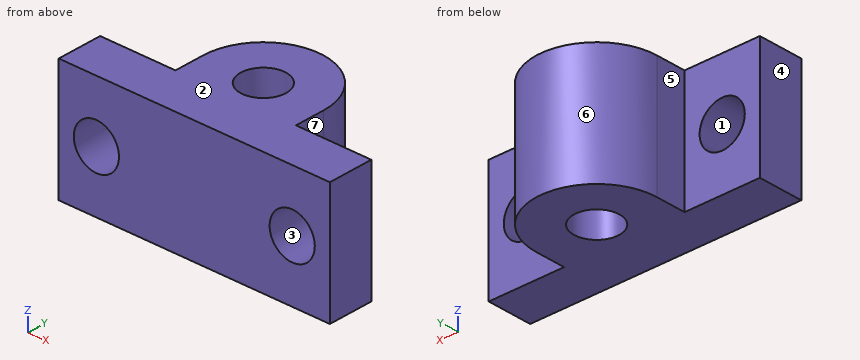
```python
from build123d import *

# Parameters (mm, degrees)
BOSS_EXTRUDE1_DEPTH = 8
SKETCH2_W           = 8
SKETCH2_H           = 3
BOSS_EXTRUDE2_DEPTH = 5
CUT_EXTRUDE1_REACH  = 18.401
SKETCH3_R           = 1.5
SKETCH4_W           = 8
SKETCH4_H           = 3
BOSS_EXTRUDE3_DEPTH = 5
CUT_EXTRUDE2_REACH  = 18.401
SKETCH5_R           = 1.5


with BuildPart() as part:
    # Sketch1 → Boss-Extrude1 (new body)
    with BuildSketch(Plane.XY):
        with BuildLine():
            ThreePointArc((8, 5), (4, 9), (0, 5))
            Line((0, 5), (2.5, 5))
            ThreePointArc((2.5, 5), (4, 6.5), (5.5, 5))
            Line((5.5, 5), (8, 5))
        make_face()
        with BuildLine():
            Line((2.5, 5), (0, 5))
            ThreePointArc((0, 5), (4, 1), (8, 5))
            Line((8, 5), (5.5, 5))
            ThreePointArc((5.5, 5), (4, 3.5), (2.5, 5))
        make_face()
        with BuildLine():
            Line((0, 5), (0, 0))
            Line((0, 0), (8, 0))
            Line((8, 0), (8, 5))
            ThreePointArc((8, 5), (4, 1), (0, 5))
        make_face()
    extrude(amount=BOSS_EXTRUDE1_DEPTH)

    # Sketch2 → Boss-Extrude2 (add)
    with BuildSketch(Plane(origin=(8, 0, 0), x_dir=(0, 0, -1), z_dir=(1, 0, 0))):
        with Locations((-4, 1.5)):
            Rectangle(SKETCH2_W, SKETCH2_H)
    extrude(amount=BOSS_EXTRUDE2_DEPTH)

    # Sketch3 → Cut-Extrude1 (cut, up to next)
    with BuildSketch(Plane(origin=(0, 3, 0), x_dir=(1, 0, 0), z_dir=(0, 1, 0)), mode=Mode.PRIVATE) as cut_extrude1_sk1:
        with Locations(Location((10.5, -4, 0), (0, 0, 270))):
            Circle(SKETCH3_R)
    cut_extrude1_tool1 = extrude(cut_extrude1_sk1.sketch, amount=-CUT_EXTRUDE1_REACH, mode=Mode.PRIVATE) & part.part
    add(cut_extrude1_tool1.solids().sort_by_distance((10.5, 3, 4))[0], mode=Mode.SUBTRACT)

    # Sketch4 → Boss-Extrude3 (add)
    with BuildSketch(Plane.ZY):
        with Locations((4, 1.5)):
            Rectangle(SKETCH4_W, SKETCH4_H)
    extrude(amount=BOSS_EXTRUDE3_DEPTH)

    # Sketch5 → Cut-Extrude2 (cut, up to next)
    with BuildSketch(Plane(origin=(0, 3, 0), x_dir=(1, 0, 0), z_dir=(0, 1, 0)), mode=Mode.PRIVATE) as cut_extrude2_sk1:
        with Locations(Location((-2.5, -4, 0), (0, 0, 180))):
            Circle(SKETCH5_R)
    cut_extrude2_tool1 = extrude(cut_extrude2_sk1.sketch, amount=-CUT_EXTRUDE2_REACH, mode=Mode.PRIVATE) & part.part
    add(cut_extrude2_tool1.solids().sort_by_distance((-2.5, 3, 4))[0], mode=Mode.SUBTRACT)


solid = part.part
```
Design review of the part built by this model. Coordinates are the model's own, in mm. Face numbers are marked on the shaded views. A direction names the side the tool comes from. Coordinates: 2 decimals unless noted, no trailing zeros. Write each loop counter-clockwise with the first axis right and the second up, starting at its lowest first coordinate (ties: lowest second). Pieces come first, ordered by that corner, then holes.
1) Add section B-B (x = 10.5). Write out the cut boundary in (y, z).
2) Insertion check: pin 1 (2.5 mm diameter, centred on x = -2.5, z = 5.5, fed in from +Y); pin 2 (4 mm diameter, centred on x = 9.5, z = 4, fed in from +Y); pin 3 (1 mm diameter, centred on y = 4.5, z = 4, fed in from -X). Each pin has a flat end and moves straight along its axis. Give the tip position at first contact, or say it passes through.
3) To check wall thickness, follow L1, parallel to Z at x = -2.5, y = 1.95; L2, parallel to X at y = 0.75, z = 3.5. State the ranges of each line that lie inside material, in increasing order.
4) Add section C-C (y = 1.5). Write out the cut boundary in (x, z).
5) Add section A-A (z = 4). Write out the cut boundary in (x, y).
6) Add section D-D (z = 7.5). Write out the cut boundary in (x, y), plus the area to 3 significant figures.
7) Mouldability with a two-part tool opening along X and no side actions: class the marked faces 1, 2, 3 and 4 as +X half, -X half, draft (parallel to the pull), parting line (faces both ways), or undercut.
8) Machinability: for the marked faces 5, 6 and 7, which of the approach directions +Z, -Z, +X, -X, +Y, -Y give a long, thin tool a straight path to every point of the face, cutting with its end or side? Answer none if there is none.
Check result:
1. outline: (0, 0) - (3, 0) - (3, 2.5) - (0, 2.5) - close; (0, 5.5) - (3, 5.5) - (3, 8) - (0, 8) - close
2. pin 1: stops at y = 3
2. pin 2: stops at y = 6.94
2. pin 3: stops at x = 0
3. L1: z = 0 to 2.5, 5.5 to 8
3. L2: x = -5 to -3.91, -1.09 to 9.09, 11.91 to 13
4. outline: (-5, 0) - (13, 0) - (13, 8) - (-5, 8) - close; hole circle Ø3 at (-2.5, 4); hole circle Ø3 at (10.5, 4)
5. outline: (-5, 0) - (-4, 0) - (-4, 3) - (-5, 3) - close; (-1, 0) - (9, 0) - (9, 3) - (8, 3) - (8, 5) arc R4 ccw to (0, 5) - (0, 3) - (-1, 3) - close; (12, 0) - (13, 0) - (13, 3) - (12, 3) - close; hole circle Ø3 at (4, 5)
6. outline: (-5, 0) - (13, 0) - (13, 3) - (8, 3) - (8, 5) arc R4 ccw to (0, 5) - (0, 3) - (-5, 3) - close; hole circle Ø3 at (4, 5)
6. area: 88.1 mm2
7. face 1: undercut
7. face 2: draft
7. face 3: undercut
7. face 4: -X half
8. face 5: +Z, -Z, -X, +Y
8. face 6: +Z, -Z, +Y
8. face 7: +Z, -Z, +X, +Y
